Geometry check sheet. Reference: the model listing, model coordinates, mm. Face numbers are marked on the shaded views. A direction names the side the tool comes from. Coordinates: 2 decimals unless noted, no trailing zeros. Write each loop counter-clockwise with the first axis right and the second up, starting at its lowest first coordinate (ties: lowest second). Pieces come first, ordered by that corner, then holes. Notation, with made-up numbers: (-6, 58) -> (7, 58) arc R12 ccw to (7, 71) -> close; hole circle Ø2 at (32.5, -34.5). An arc over 180 degrees is marked (long way). Answer in a Markdown table with one row per item. Add a question column.
1. Mould release check, pull along X, two halves, no side actions. Record for the marked faces 3, 4, 5 and 6: pulls with the +X half, pulls with the -X half, needs draft (parallel to the pull), parting line crosses it, or undercut.
2. Scan lines: L1, parallel to X at y = 399, z = 358; L2, parallel to Z at x = 332, y = 279; L3, parallel to Y at x = 557, z = 415.5. Record each from-to range of solid material in increasing order. Write a range as from..to.
3. Cross-section at A-A on y = 453. Record the cut outline in (x, z), and give its area (3 significant figures).
4. Set-up check for the marked faces 1 and 2: record each of +Z, -Z, +X, -X, +Y, -Y from which the full face is reachable in a straight line by a thin tool's end or side.
5. Depth check by flat-ended pin: P1, Ø5, axis at x = 399, z = 181, coming from the -Y side. Enter the tip coordinate at first touch or a pass-through.
6. Cross-section at C-C on z = 246.5. Record the cut outline in (x, y).
7. Cross-section at B-B on x = 551. Record the cut outline in (y, z), and give its area (4 significant figures).
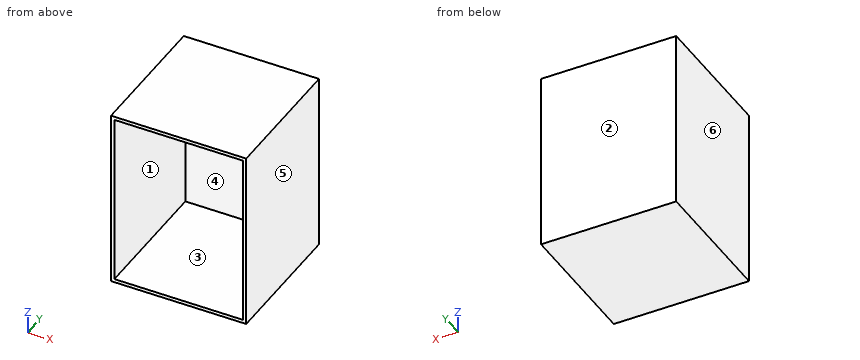
```python
from build123d import *

# Parameters (mm, degrees)
F0_W     = 600
F0_H     = 800
F1_DEPTH = 600
F2_T     = -15


with BuildPart() as f1:
    # F0 (on Right) → F1 (new body)
    with BuildSketch(Plane.YZ):
        with Locations((300, 400)):
            Rectangle(F0_W, F0_H)
    extrude(amount=F1_DEPTH)

    # F2
    f2_openings = [f1.faces().sort_by_distance(p)[0] for p in [
        (300, 0, 400),
    ]]
    offset(amount=F2_T, openings=f2_openings)


with BuildPart() as f3_1:
    # F3: copy of F1
    add(f1.part.moved(Location((700, 0, 0))))


solid = f1.part
```
Results found:
| question | item | result |
|---|---|---|
| 1 | face 3 | undercut |
| 1 | face 4 | undercut |
| 1 | face 5 | pulls with the +X half |
| 1 | face 6 | pulls with the -X half |
| 2 | L1 | x = 0..15, 585..600 |
| 2 | L2 | z = 0..15, 785..800 |
| 2 | L3 | y = 585..600 |
| 3 | outline | (0, 0) -> (600, 0) -> (600, 800) -> (0, 800) -> close; hole (15, 15) -> (585, 15) -> (585, 785) -> (15, 785) -> close |
| 3 | area | 41,100 mm^2 |
| 4 | face 1 | -Y |
| 4 | face 2 | +Z, -Z, +X, -X, +Y |
| 5 | P1 | stops at y = 585 |
| 6 | outline | (0, 0) -> (15, 0) -> (15, 585) -> (585, 585) -> (585, 0) -> (600, 0) -> (600, 600) -> (0, 600) -> close |
| 7 | outline | (0, 0) -> (600, 0) -> (600, 800) -> (0, 800) -> (0, 785) -> (585, 785) -> (585, 15) -> (0, 15) -> close |
| 7 | area | 29,550 mm^2 |
